```python
from build123d import *

# Parameters (mm, degrees)
SKETCH_1_R          = 5.5
EXTRUDE_1_DEPTH     = 2
SKETCH_4_R          = 6.25
EXTRUDE_2_DEPTH     = 1
SKETCH_2_R          = 2
CUT_EXTRUDE_1_DEPTH = 10.701803956
SKETCH_3_R          = 4.6
SKETCH_3_R_2        = 2.79
CUT_EXTRUDE_2_DEPTH = 0.2


with BuildPart() as part:
    # 草圖1 → 填料-伸長1 (new, symmetric)
    with BuildSketch(Plane.XY):
        Circle(SKETCH_1_R)
    extrude(amount=EXTRUDE_1_DEPTH, both=True)

    # 草圖4 → 填料-伸長2 (add)
    with BuildSketch(Plane(origin=(0, 0, -2), x_dir=(-1, 0, 0), z_dir=(0, 0, -1))):
        Circle(SKETCH_4_R)
    extrude(amount=-EXTRUDE_2_DEPTH)

    # 草圖2 → 除料-伸長1 (cut, through all)
    with BuildSketch(Plane.XY.offset(2)):
        Circle(SKETCH_2_R)
    extrude(amount=-CUT_EXTRUDE_1_DEPTH, mode=Mode.SUBTRACT)

    # 草圖3 → 除料-伸長2 (cut)
    with BuildSketch(Plane.XY.offset(2)):
        Circle(SKETCH_3_R)
        Circle(SKETCH_3_R_2, mode=Mode.SUBTRACT)
    cut_extrude_2 = extrude(amount=-CUT_EXTRUDE_2_DEPTH, mode=Mode.SUBTRACT)

    # 鏡射1: 除料-伸長2 across plane
    add(cut_extrude_2.mirror(Plane.XY), mode=Mode.SUBTRACT)


solid = part.part
```
Model file for the job. Use its own axes, mm. A direction names the side the tool comes from. Give positions to 0.01 mm unless a question says otherwise; leave off trailing zeros. Write each loop counter-clockwise with the first axis right and the second up, starting at its lowest first coordinate (ties: lowest second). Pieces come first, ordered by that corner, then holes. Notation, with made-up numbers: (6, 53.25) - (56, 53.25) arc R18 ccw to (56, 61.25) - close; hole circle Ø6 at (36.5, 15). An arc over 180 degrees is marked (long way). One line per question, with ' | ' between items. Start each with the question number.
(1) 3-axis set-ups, long thin cutter, end or side, ignore diameter. For faces 4 (the face through (0, -2, 0)), 5 (the face through (0, -3, -1.8)), 6 (the face through (-1.19, -5.37, 0.52)): which of +Z, -Z, +X, -X, +Y, -Y reach the whole face in a straight line?
(2) Slice it at A-A on y = 0. Write the cut outline in (x, z), plus the area to 3 significant figures.
(3) Pin check, flat tip, straight feed: P1, Ø1, axis at x = 4.5, z = -1, coming from the +Y side. Stop position of the tip, or through.
(4) Wall check: line 1 along Y through (x, z) = (0, 1.9); line 2 along Y through (x, z) = (0, 1.25); line 3 along Z through (x, y) = (-1.75, -3.75). Give the ranges that are in metal, low to high. Write a range as from..to.
(5) Two-plate mould, pull along Y, no slides. Class faces 1 (the face through (0, -3, 1.8)), 2 (the face through (3, -4, 2)), 3 (the face through (-5.96, 1.88, -1.51)): +Y half, -Y half, draft (parallel to the pull), parting line (faces both ways), or undercut.
(6) Slice it at D-D on y = 2.5. Write the cut outline in (x, z), plus the area to 3 significant figures.
(7) Slice it at C-C on z = 1. Write the cut outline in (x, y).
Results below:
1) face 4: +Z, -Z | face 5: -Z | face 6: +Z
2) outline: (-6.25, -2) - (-4.6, -2) - (-4.6, -1.8) - (-2.79, -1.8) - (-2.79, -2) - (-2, -2) - (-2, 2) - (-2.79, 2) - (-2.79, 1.8) - (-4.6, 1.8) - (-4.6, 2) - (-5.5, 2) - (-5.5, -1) - (-6.25, -1) - close; (2, -2) - (2.79, -2) - (2.79, -1.8) - (4.6, -1.8) - (4.6, -2) - (6.25, -2) - (6.25, -1) - (5.5, -1) - (5.5, 2) - (4.6, 2) - (4.6, 1.8) - (2.79, 1.8) - (2.79, 2) - (2, 2) - close | area: 28.1 mm^2
3) P1: y = 4.8
4) line 1: -5.5..-4.6, -2.79..-2, 2..2.79, 4.6..5.5 | line 2: -5.5..-2, 2..5.5 | line 3: -1.8..1.8
5) face 1: undercut | face 2: draft | face 3: parting line
6) outline: (-5.73, -2) - (-3.86, -2) - (-3.86, -1.8) - (-1.24, -1.8) - (-1.24, -2) - (1.24, -2) - (1.24, -1.8) - (3.86, -1.8) - (3.86, -2) - (5.73, -2) - (5.73, -1) - (4.9, -1) - (4.9, 2) - (3.86, 2) - (3.86, 1.8) - (1.24, 1.8) - (1.24, 2) - (-1.24, 2) - (-1.24, 1.8) - (-3.86, 1.8) - (-3.86, 2) - (-4.9, 2) - (-4.9, -1) - (-5.73, -1) - close | area: 38.8 mm^2
7) outline: circle Ø11 at (0, 0); hole circle Ø4 at (0, 0)
